Here's how the part is built. I have some questions about the finished solid (model axes, mm). Face numbers are marked on the shaded views. A direction names the side the tool comes from. Coordinates: 2 decimals unless noted, no trailing zeros. Write each loop counter-clockwise with the first axis right and the second up, starting at its lowest first coordinate (ties: lowest second). Pieces come first, ordered by that corner, then holes.
(1) For pin 1 Ø3 at (x, y) = (12, 15.5) entering from -Z; pin 2 Ø4 at (y, z) = (6, -23.47) entering from -X; pin 3 Ø1.8 at (y, z) = (5, -24) entering from +X, each with a flat end and sliding along its axis, tell me the tip position at first contact or that it passes through.
(2) Imagine slicing it at B-B, the plane z = -12. List the corners of the cut face in (x, y) for me.
(3) Imagine slicing it at A-A, the plane x = -28. List the corners of the cut face in (y, z) for me.
(4) Please list where these lines run through material, in increasing order: probe 1 along X at (y, z) = (1.75, -21); probe 2 along Y at (x, z) = (25.5, -23.5); probe 3 along Y at (x, z) = (33, -22.25).
(5) Thinking about a two-plate mould opening in Z: for the marked faces 3, 4 and 5, which applies, released by +Z, released by -Z, zero draft, split by the parting line, or undercut?
(6) Imagine slicing it at C-C, the plane y = 14.25. List the corners of the cut face in (x, z) for me, plus the area to 3 significant figures.
(7) Imagine slicing it at D-D, the plane z = -4.75. List the corners of the cut face in (x, y) for me.
(8) Which directions (+Z, -Z, +X, -X, +Y, -Y) give clear straight access to the entire face, cutting with the end or side of a thin tool? Please do the marked faces 1 and 2.
```python
from build123d import *

# Parameters (mm, degrees)
SKETCH_1_R                = 8
EXTRUDE_1_DEPTH           = 25
SKETCH_2_W                = 2
SKETCH_2_H                = 7.062746067
CUT_EXTRUDE_1_DEPTH       = 56.839054433
HOLE_START                = -42
HOLE_WIZARD_1_OUTLINE_R   = 3
HOLE_WIZARD_1_DEPTH       = 3.4
HOLE_START_2              = -38.6
HOLE_WIZARD_1_2_OUTLINE_R = 1.6
HOLE_WIZARD_1_2_DEPTH     = 7.6
HOLE_WIZARD_M3_1_D        = 2.5
HOLE_WIZARD_M3_1_DEPTH    = 11.001


# Read off the part's stored shape, not the designer's step: 打孔尺寸(%根据)内六角圆柱头螺钉的类型1
with BuildPart() as part:
    # 草图1 → 凸台-拉伸1 (new body)
    with BuildSketch(Plane(origin=(0, 0, 0), x_dir=(1, 0, 0), z_dir=(0, 1, 0))):
        Polygon((-18, 27), (-18, 7), (18, 7), (18, 27), (42, 27), (42, 0), (-42, 0), (-42, 27), align=None)
        with Locations(Location((-30, 12, 0), (0, 0, 270))):
            Circle(SKETCH_1_R, mode=Mode.SUBTRACT)
        with Locations(Location((30, 12, 0), (0, 0, 90))):
            Circle(SKETCH_1_R, mode=Mode.SUBTRACT)
    extrude(amount=EXTRUDE_1_DEPTH)

    # 草图2 → 切除-拉伸1 (cut, through all)
    with BuildSketch(Plane(origin=(0, 25, 0), x_dir=(1, 0, 0), z_dir=(0, 1, 0))):
        with Locations((-30, 23.468626967)):
            Rectangle(SKETCH_2_W, SKETCH_2_H)
    cut_extrude_1 = extrude(amount=-CUT_EXTRUDE_1_DEPTH, mode=Mode.SUBTRACT)

    # 打孔尺寸(%根据)内六角圆柱头螺钉的类型1 outline → 打孔尺寸(%根据)内六角圆柱头螺钉的类型1 (cut)
    with BuildSketch(Plane.YZ.offset(HOLE_START)):
        with Locations((6, -23.468626967)):
            Circle(HOLE_WIZARD_1_OUTLINE_R)
        with Locations((19, -23.468626967)):
            Circle(HOLE_WIZARD_1_OUTLINE_R)
    hole_wizard_1 = extrude(amount=HOLE_WIZARD_1_DEPTH, mode=Mode.SUBTRACT)

    # Hole Wizard 1 2 outline → Hole Wizard 1 2 (cut)
    with BuildSketch(Plane.YZ.offset(HOLE_START_2)):
        with Locations((6, -23.468626967)):
            Circle(HOLE_WIZARD_1_2_OUTLINE_R)
        with Locations((19, -23.468626967)):
            Circle(HOLE_WIZARD_1_2_OUTLINE_R)
    hole_wizard_1_2 = extrude(amount=HOLE_WIZARD_1_2_DEPTH, mode=Mode.SUBTRACT)

    # M3 螺纹孔1
    with Locations(Plane(origin=(-18, 0, 0), x_dir=(0, 0, -1), z_dir=(1, 0, 0))):
        with Locations((23.468626967, 19), (23.468626967, 6)):
            hole_wizard_m3_1 = Hole(HOLE_WIZARD_M3_1_D / 2, depth=HOLE_WIZARD_M3_1_DEPTH)

    # 镜向1: 切除-拉伸1, 打孔尺寸(%根据)内六角圆柱头螺钉的类型1, Hole Wizard 1 2, M3 螺纹孔1 across plane
    add(cut_extrude_1.mirror(Plane(origin=(0, 0, 0), x_dir=(0, 0, 1), z_dir=(1, 0, 0))), mode=Mode.SUBTRACT)
    add(hole_wizard_1.mirror(Plane(origin=(0, 0, 0), x_dir=(0, 0, 1), z_dir=(1, 0, 0))), mode=Mode.SUBTRACT)
    add(hole_wizard_1_2.mirror(Plane(origin=(0, 0, 0), x_dir=(0, 0, 1), z_dir=(1, 0, 0))), mode=Mode.SUBTRACT)
    add(hole_wizard_m3_1.mirror(Plane(origin=(0, 0, 0), x_dir=(0, 0, 1), z_dir=(1, 0, 0))), mode=Mode.SUBTRACT)


solid = part.part
```
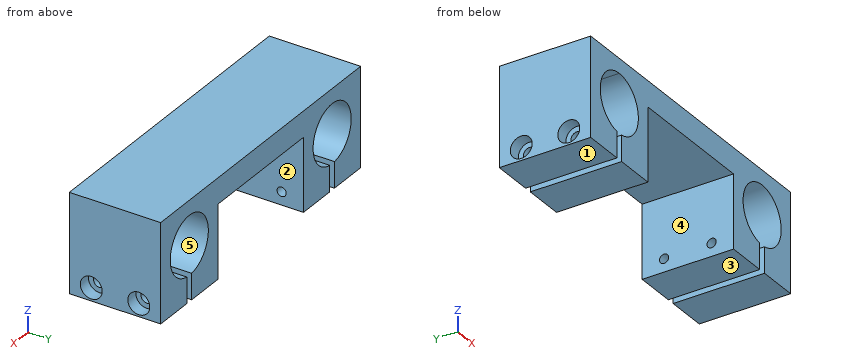
Recorded:
1. pin 1: stops at z = -7
1. pin 2: stops at x = -38.6
1. pin 3: stops at x = 38.6
2. outline: (-42, 0) - (-38, 0) - (-38, 25) - (-42, 25) - close; (-22, 0) - (-18, 0) - (-18, 25) - (-22, 25) - close; (18, 0) - (22, 0) - (22, 25) - (18, 25) - close; (38, 0) - (42, 0) - (42, 25) - (38, 25) - close
3. outline: (0, -27) - (25, -27) - (25, -19.75) - (0, -19.75) - close; (0, -4.25) - (25, -4.25) - (25, 0) - (0, 0) - close; hole circle Ø2.5 at (6, -23.47); hole circle Ø2.5 at (19, -23.47)
4. probe 1: x = -42 to -31, -29 to -18, 18 to 29, 31 to 42
4. probe 2: y = 0 to 4.75, 7.25 to 17.75, 20.25 to 25
4. probe 3: y = 0 to 4.96, 7.04 to 17.96, 20.04 to 25
5. face 3: released by -Z
5. face 4: zero draft
5. face 5: undercut
6. outline: (-42, -27) - (-31, -27) - (-31, -19.94) arc R8 cw (long way) to (-29, -19.94) - (-29, -27) - (-18, -27) - (-18, -7) - (18, -7) - (18, -27) - (29, -27) - (29, -19.94) arc R8 cw (long way) to (31, -19.94) - (31, -27) - (42, -27) - (42, 0) - (-42, 0) - close
6. area: 1,120 mm2
7. outline: (-42, 0) - (-33.38, 0) - (-33.38, 25) - (-42, 25) - close; (-26.62, 0) - (26.62, 0) - (26.62, 25) - (-26.62, 25) - close; (33.38, 0) - (42, 0) - (42, 25) - (33.38, 25) - close
8. face 1: -Z, +X, -X, +Y, -Y
8. face 2: -Z, +Y, -Y
